Can you work these out from the model? Positions are in its coordinate system, mm. A direction names the side the tool comes from. Give positions to 0.01 mm unless a question says otherwise; leave off trailing zeros. Order: outer loops, then holes, each group sorted by start corner. A loop starts at its lowest first (then second) coordinate and runs counter-clockwise, first axis right, second up.
Item 1: I want a section at A-A, the plane z = 12. Write out the boundary of the cut face in (x, y), then the cut area to 3 significant figures.
Item 2: I'm going to push flat-ended pins straight in: pin 1 Ø2.5 at (y, z) = (6.5, 8) entering from -X; pin 2 Ø2 at (y, z) = (4.5, 10.5) entering from -X; pin 3 Ø2.5 at (y, z) = (7, 10) entering from -X; pin 4 Ø4 at (y, z) = (6.975, 10) entering from +X. Where does each tip first touch, or does it pass through?
Item 3: If we mould it in two halves opening along Y, with no side actions, what happens to faces 4 (the cylindrical face through (4.623, 9.415, 17.277)), 5 (the flat face through (0.375, 6, 12)), 6 (the flat face through (2.375, 5.6, 8.7))? For each: +Y half, -Y half, draft (parallel to the pull), parting line (faces both ways), or undercut.
Item 4: If I drill on line 1 along X through (y, z) = (0, 8); line 2 along Y through (x, z) = (0.5, 9.25); line 3 along X through (y, z) = (-2.75, 4.5), over which ranges is the centre line in solid material (lowest first)?
Item 5: Which directions (+Z, -Z, +X, -X, +Y, -Y) give clear straight access to the entire face, cutting with the end or side of a thin tool? Please do faces 1 (the cylindrical face through (-0.63, 11.73, 10.04)), 2 (the cylindrical face through (0.646, 9.333, 17.304)), 3 (the flat face through (-4.07, 5.61, 7.69)).
Item 6: I want a section at B-B, the plane z = 7.75. Write out the boundary of the cut face in (x, y), then the cut area to 3 significant figures.
```python
from build123d import *

# Parameters (mm, degrees)
EXTRUDE002_DEPTH     = 10
SKETCH004_R          = 3.1
EXTRUDE001_DEPTH     = 10
EXTRUDE_DEPTH        = 20
SKETCH001_R          = 4.1
POCKET_DEPTH         = 10
POCKET001_DEPTH      = 10
SKETCH003_R          = 1.55
POCKET002_DEPTH      = 6.126038
POCKET002_DEPTH_BACK = -6.875962
CHAMFER_SIZE         = 5
FILLET_R             = 5
FILLET001_R          = 0.9


with BuildPart() as extrude002:
    # Sketch005 → Extrude002 (new body)
    with BuildSketch(Plane.YZ.offset(-0.375038)):
        Polygon((9.659679, 11.55), (6.975, 13.1), (4.290321, 11.55), (4.290321, 8.45), (6.975, 6.9), (9.659679, 8.45), align=None)
    extrude(amount=-EXTRUDE002_DEPTH)


with BuildPart() as extrude002_1:
    # Extrude002 placement: moved
    add(extrude002.part.moved(Location((-2, 0, 0))))


with BuildPart() as extrude001:
    # Sketch004 → Extrude001 (new body)
    with BuildSketch(Plane(origin=(0.374962, 0, 0), x_dir=(0, -1, 0), z_dir=(-1, 0, 0))):
        with Locations((-6.975, 10)):
            Circle(SKETCH004_R)
    extrude(amount=-EXTRUDE001_DEPTH)


with BuildPart() as extrude001_1:
    # Extrude001 placement: moved
    add(extrude001.part.moved(Location((2, 0, 0))))


with BuildPart() as fillet001:
    # Sketch → Extrude (new body)
    with BuildSketch(Plane.XY):
        with BuildLine():
            Line((-0.375038, 12), (-0.375038, 0))
            Line((-0.375038, 0), (0.374962, 0))
            Line((0.374962, 0), (0.374962, 12))
            Line((0.374962, 12), (4.374962, 12))
            Line((4.374962, 12), (6.389918, 1.191196))
            ThreePointArc((-6.389921, 1.191182), (7e-06, -6.5), (6.389918, 1.191196))
            Line((-4.375038, 12), (-6.389921, 1.191182))
            Line((-0.375038, 12), (-4.375038, 12))
        make_face()
    extrude(amount=EXTRUDE_DEPTH)

    # Sketch001 → Pocket (cut)
    with BuildSketch(Plane(origin=(0, 0, 0), x_dir=(1, 0, 0), z_dir=(0, 0, -1))):
        Circle(SKETCH001_R)
    extrude(amount=-POCKET_DEPTH, mode=Mode.SUBTRACT)

    # Sketch002 → Pocket001 (cut)
    with BuildSketch(Plane.XY.offset(20)):
        with BuildLine():
            ThreePointArc((-1.719738, 1.95), (0, -2.6), (1.719738, 1.95))
            Line((-1.719738, 1.95), (1.719738, 1.95))
        make_face()
    extrude(amount=-POCKET001_DEPTH, mode=Mode.SUBTRACT)

    # Sketch003 → Pocket002 (cut, two sides)
    with BuildSketch(Plane(origin=(0.374962, 0, 0), x_dir=(0, -1, 0), z_dir=(-1, 0, 0))) as pocket002_sk:
        with Locations((-6.975, 10)):
            Circle(SKETCH003_R)
    extrude(amount=-POCKET002_DEPTH, mode=Mode.SUBTRACT)
    extrude(pocket002_sk.sketch, amount=-POCKET002_DEPTH_BACK, mode=Mode.SUBTRACT)

    # Cut: cut Extrude001
    add(extrude001_1.part, mode=Mode.SUBTRACT)

    # Cut001: cut Extrude002
    add(extrude002_1.part, mode=Mode.SUBTRACT)

    # Chamfer
    chamfer_edges = [fillet001.edges().sort_by_distance(p)[0] for p in [
        (-2.375038, 12, 0),
        (2.374962, 12, 0),
        (-2.375038, 12, 20),
        (2.374962, 12, 20),
    ]]
    chamfer(chamfer_edges, length=CHAMFER_SIZE)

    # Fillet
    fillet_edges = [fillet001.edges().sort_by_distance(p)[0] for p in [
        (-2.841066, 7, 0),
        (2.841007, 7, 0),
        (-2.375038, 12, 5),
        (-2.375038, 12, 15),
        (-2.841066, 7, 20),
        (2.841007, 7, 20),
        (2.374962, 12, 5),
        (2.374962, 12, 15),
    ]]
    fillet(fillet_edges, radius=FILLET_R)

    # Fillet001
    fillet001_edges = [fillet001.edges().sort_by_distance(p)[0] for p in [
        (-0.375038, 3.439466, 20),
        (-1.047388, 1.95, 20),
        (-6.041542, 3.060057, 20),
        (7e-06, -6.5, 20),
        (6.041527, 3.060064, 20),
        (0, -2.6, 20),
        (0.374962, 3.439466, 20),
        (1.04735, 1.95, 20),
    ]]
    fillet(fillet001_edges, radius=FILLET001_R)


solid = fillet001.part
```
Results list:
1. outline: (-6.39, 1.19) arc R6.5 ccw (long way) to (6.39, 1.19) - (5.75, 4.61) - (2.37, 4.61) - (2.37, 9.34) - (4.87, 9.34) - (4.51, 11.26) arc R0.9 ccw to (3.63, 12) - (1.27, 12) arc R0.9 ccw to (0.37, 11.1) - (0.37, 1.95) - (1.72, 1.95) arc R2.6 cw (long way) to (-1.72, 1.95) - (-0.38, 1.95) - (-0.38, 11.1) arc R0.9 ccw to (-1.28, 12) - (-3.63, 12) arc R0.9 ccw to (-4.51, 11.26) - (-4.96, 8.88) - (-2.38, 8.88) - (-2.38, 5.07) - (-5.67, 5.07) - close
1. area: 145 mm2
2. pin 1: stops at x = -5.63
2. pin 2: stops at x = -5.96
2. pin 3: passes through
2. pin 4: stops at x = 2.37
3. face 4: +Y half
3. face 5: draft
3. face 6: undercut
4. line 1: x = -6.5 to -4.1, 4.1 to 6.5
4. line 2: y = -6.48 to -4.07, 4.07 to 5.62, 8.33 to 11.56
4. line 3: x = -5.89 to -3.04, 3.04 to 5.89
5. face 1: +Z, -Z, +Y
5. face 2: +Z, +Y
5. face 3: -X
6. outline: (-6.39, 1.19) arc R6.5 ccw (long way) to (6.39, 1.19) - (5.71, 4.84) - (2.37, 4.84) - (2.37, 9.11) - (4.91, 9.11) - (4.51, 11.26) arc R0.9 ccw to (3.63, 12) - (1.27, 12) arc R0.9 ccw to (0.37, 11.1) - (0.37, 4.08) arc R4.1 cw (long way) to (-0.38, 4.08) - (-0.38, 11.1) arc R0.9 ccw to (-1.28, 12) - (-3.63, 12) arc R0.9 ccw to (-4.51, 11.26) - (-5.04, 8.45) - (-2.38, 8.45) - (-2.38, 5.5) - (-5.59, 5.5) - close
6. area: 118 mm2
